Design review of the part built by this model. Coordinates are the model's own, in mm. Face numbers are marked on the shaded views. Give positions to 0.01 mm unless a question says otherwise; leave off trailing zeros. Order: outer loops, then holes, each group sorted by start corner. A loop starts at its lowest first (then second) coordinate and runs counter-clockwise, first axis right, second up. Notation, with made-up numbers: (78.25, 17.25) -> (125.25, 17.25) arc R22 ccw to (125.25, 24.25) -> close; hole circle Ø5 at (34.25, 63). An arc over 180 degrees is marked (long way). One line per item, written item: value. Start each with the question number.
1) For pin 1 (2 mm diameter, centred on y = 11.5, z = 13.5, fed in from +X); pin 2 (12 mm diameter, centred on x = -10, y = 13, fed in from -Z); pin 3 (3 mm diameter, centred on x = -29.5, y = 7, fed in from +Z), all flat-tipped, find the tip position at first contact; note any pin that passes through.
2) The part is to be moulded in two halves that separate along X. For the marked faces 1, 2 and 3, say which applies: released by +X, released by -X, zero draft, split by the parting line, or undercut.
3) Consider section B-B (y = 18). State the section outline as (x, z) points, plus the area to 3 significant figures.
4) Consider section A-A (x = 0). State the section outline as (y, z) points.
5) Wall thickness on line 1 along X through (y, z) = (11.75, 0); line 2 along Y through (x, z) = (42, -23); line 3 along X through (y, z) = (1.5, -36): over which ranges is each line inside the solid? List them lowest first. Write a range as from..to.
6) Consider section C-C (x = 24). State how many separate pieces and enclosed holes the cut face has, plus the area to 3 significant figures.
from build123d import *

# Parameters (mm, degrees)
SKETCH_2_R               = 7
CUT_EXTRUDE_1_DEPTH      = 89.18163074
PATTERN_CIRCULAR_1_COUNT = 6


with BuildPart() as part:
    # 草图1 → 旋转1 (revolve)
    with BuildSketch(Plane.XY, mode=Mode.PRIVATE) as revolve_1_sk:
        Polygon((20, 0), (58, 0), (60, 2), (60, 14), (58, 16), (35, 16), (35, 24), (20, 24), align=None)
    revolve(revolve_1_sk.sketch.rotate(Axis((0, -10, 0), (0, 1, 0)), 90), axis=Axis((0, -10, 0), (0, 1, 0)))

    # 草图2 → 切除-拉伸1 (cut, through all)
    with BuildSketch(Plane(origin=(0, 0, 0), x_dir=(1, 0, 0), z_dir=(0, 1, 0))):
        with Locations(Location((45, 0, 0), (0, 0, 270))):
            Circle(SKETCH_2_R)
    cut_extrude_1 = extrude(amount=CUT_EXTRUDE_1_DEPTH, mode=Mode.SUBTRACT)

    # 阵列(圆周)1: 切除-拉伸1 ×6 about axis
    pattern_circular_1_axis = Axis((0, 0, 0), (0, 1, 0))
    for i in range(1, PATTERN_CIRCULAR_1_COUNT):
        add(cut_extrude_1.rotate(pattern_circular_1_axis, i * 360 / PATTERN_CIRCULAR_1_COUNT), mode=Mode.SUBTRACT)


solid = part.part
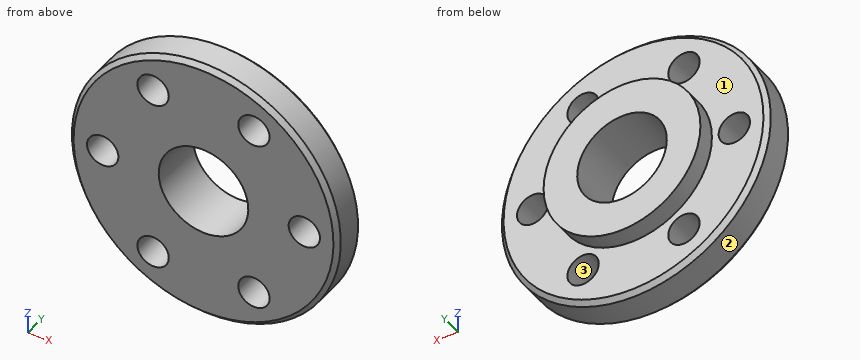
Checked values:
1. pin 1: stops at x = 58.68
1. pin 2: stops at z = -59.87
1. pin 3: stops at z = 53.07
2. face 1: zero draft
2. face 2: split by the parting line
2. face 3: undercut
3. outline: circle Ø70 at (0, 0); hole circle Ø40 at (0, 0)
3. area: 2,590 mm^2
4. outline: (0, -58) -> (2, -60) -> (14, -60) -> (16, -58) -> (16, -35) -> (24, -35) -> (24, -20) -> (0, -20) -> close; (0, 20) -> (24, 20) -> (24, 35) -> (16, 35) -> (16, 58) -> (14, 60) -> (2, 60) -> (0, 58) -> close
5. line 1: x = -60..-52, -38..-20, 20..38, 52..60
5. line 2: y = 0..16
5. line 3: x = -47.37..-28.84, -16.16..16.16, 28.84..47.37
6. separate pieces: 3
6. enclosed holes: 0
6. area: 1,720 mm^2
